Input: part model. Units: mm. Frame: model coordinates. Coordinates: 2 decimals unless noted, no trailing zeros. Write each loop counter-clockwise with the first axis right and the second up, starting at its lowest first coordinate (ties: lowest second). Pieces come first, ordered by that corner, then holes.
1) Section query A-A (x = 0). Output: boundary loops of the cut face in (y, z), then the cut area to 3 significant figures.
2) Pin query (flat end, axial travel): pin 1 Ø4 at (y, z) = (7, -11) entering from +X. Return the tip coordinate at first contact, or that it passes through.
3) Section query B-B (z = 0). Output: boundary loops of the cut face in (x, y).
4) Line query: L1, parallel to Z at x = -21, y = 3.5; L2, parallel to X at y = 6, z = 21; L3, parallel to X at y = 1.75, z = 19. Output: solid intervals per line, ascending.
5) Section query C-C (y = 2). State how many separate pieces and enclosed holes the cut face has, then the cut area to 3 significant figures.
from build123d import *

# Parameters (mm, degrees)
BASE_PLATE_BOSS_EXTRUDE1_DEPTH                 = 25
BASE_PLATE_BOSS_EXTRUDE1_DEPTH_BACK            = 25
SKETCH5_R                                      = 5
SHAFT_CUT_EXTRUDE1_DEPTH                       = 8
SKETCH6_R                                      = 8
SHAFT_BEARING_CUT_EXTRUDE2_DEPTH               = 2.5
SKETCH7_R                                      = 1.5
BEARING_PLATE_MOUNTING_HOLES_CUT_EXTRUDE_DEPTH = 8
SKETCH8_R                                      = 1.5
BASE_SIDE_MOUNTING_HOLES_CUT_EXTRUDE4_DEPTH    = 8


with BuildPart() as part:
    # Sketch3 → Base Plate Boss-Extrude1 (new, two sides: drawn at the far end of the back side and taken through both)
    with BuildSketch(Plane.XY.offset(-BASE_PLATE_BOSS_EXTRUDE1_DEPTH_BACK)):
        Polygon((90.858272566, 8), (91.670882932, 0), (-91.670882932, 0), (-90.858272566, 8), align=None)
    extrude(amount=BASE_PLATE_BOSS_EXTRUDE1_DEPTH + BASE_PLATE_BOSS_EXTRUDE1_DEPTH_BACK)

    # Sketch4 → Base Plate Chassi Rounding Cut-Revolve1 (revolve, cut)
    with BuildSketch(Plane.XY):
        Polygon((90.858272566, 8), (91.670882932, 0), (97.920865853, 0), (97.920865853, 8), (91.670882932, 8), align=None)
    revolve(axis=Axis((0, 0, 0), (0, 1, 0)), mode=Mode.SUBTRACT)

    # Sketch5 → Shaft Cut-Extrude1 (cut)
    with BuildSketch(Plane.XZ):
        Circle(SKETCH5_R)
    extrude(amount=-SHAFT_CUT_EXTRUDE1_DEPTH, mode=Mode.SUBTRACT)

    # Sketch6 → Shaft Bearing Cut-Extrude2 (cut)
    with BuildSketch(Plane(origin=(0, 8, 0), x_dir=(1, 0, 0), z_dir=(0, 1, 0))):
        with Locations(Location((0, 0, 0), (0, 0, 180))):
            Circle(SKETCH6_R)
    extrude(amount=-SHAFT_BEARING_CUT_EXTRUDE2_DEPTH, mode=Mode.SUBTRACT)

    # Sketch7 → Bearing Plate Mounting Holes Cut-Extrude3 (cut)
    with BuildSketch(Plane(origin=(0, 8, 0), x_dir=(1, 0, 0), z_dir=(0, 1, 0))):
        with Locations(Location((12, 20, 0), (0, 0, 180))):
            Circle(SKETCH7_R)
        with Locations(Location((-12, 20, 0), (0, 0, 180))):
            Circle(SKETCH7_R)
        with Locations(Location((-12, -20, 0), (0, 0, 180))):
            Circle(SKETCH7_R)
        with Locations(Location((12, -20, 0), (0, 0, 180))):
            Circle(SKETCH7_R)
    extrude(amount=-BEARING_PLATE_MOUNTING_HOLES_CUT_EXTRUDE_DEPTH, mode=Mode.SUBTRACT)

    # Sketch8 → Base Side Mounting Holes Cut-Extrude4 (cut)
    with BuildSketch(Plane(origin=(0, 8, 0), x_dir=(1, 0, 0), z_dir=(0, 1, 0))):
        with Locations(Location((21, 20, 0), (0, 0, 180))):
            Circle(SKETCH8_R)
        with Locations(Location((-21, 20, 0), (0, 0, 180))):
            Circle(SKETCH8_R)
        with Locations(Location((-21, -20, 0), (0, 0, 180))):
            Circle(SKETCH8_R)
        with Locations(Location((21, -20, 0), (0, 0, 180))):
            Circle(SKETCH8_R)
    extrude(amount=-BASE_SIDE_MOUNTING_HOLES_CUT_EXTRUDE4_DEPTH, mode=Mode.SUBTRACT)


solid = part.part
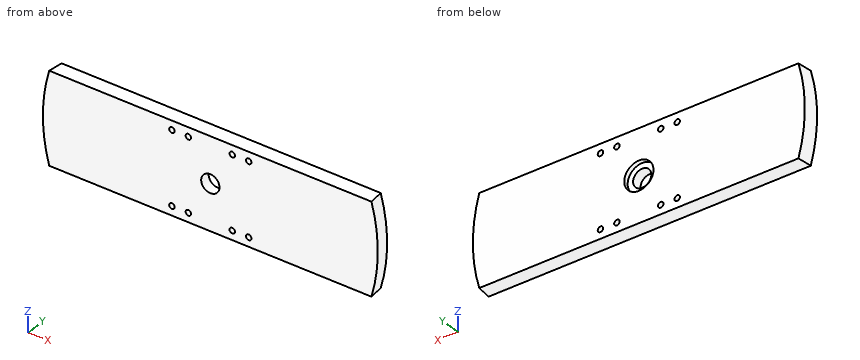
Answer:
1. outline: (0, -25) - (8, -25) - (8, -8) - (5.5, -8) - (5.5, -5) - (0, -5) - close; (0, 5) - (5.5, 5) - (5.5, 8) - (8, 8) - (8, 25) - (0, 25) - close
1. area: 305 mm2
2. pin 1: stops at x = 90.6
3. outline: (-91.67, 0) - (-5, 0) - (-5, 5.5) - (-8, 5.5) - (-8, 8) - (-90.86, 8) - close; (5, 0) - (91.67, 0) - (90.86, 8) - (8, 8) - (8, 5.5) - (5, 5.5) - close
4. L1: z = -25 to -21.5, -18.5 to 18.5, 21.5 to 25
4. L2: x = -88.61 to -22.12, -19.88 to -13.12, -10.88 to 10.88, 13.12 to 19.88, 22.12 to 88.61
4. L3: x = -89.5 to -22.12, -19.88 to -13.12, -10.88 to 10.88, 13.12 to 19.88, 22.12 to 89.5
5. separate pieces: 1
5. enclosed holes: 9
5. area: 8,900 mm2
